Autodesk Inventor part; units mm, degrees
ref_plane "YZ Plane" through (0, 0, 0) normal (1, 0, 0) x (0, 1, 0)
ref_plane "XZ Plane" through (0, 0, 0) normal (0, 1, 0) x (-1, 0, 0)
ref_plane "XY Plane" through (0, 0, 0) normal (0, 0, 1) x (1, 0, 0)
sketch "Sketch1" plane through (0, 0, 0) normal (0, 1, 0) x (-1, 0, 0)
  circle A0 centre (0, 15.6484) radius 5.5
  line L0 (0, 15.6484) -> (0, -0.3516)
  circle A1 centre (0, -0.3516) radius 5.5
  circle A2 centre (0, 15.6484) radius 2.5
  circle A3 centre (0, -0.3516) radius 2.5
  line L1 (5.5, 15.6484) -> (5.5, -0.3516)
  line L2 (-5.5, 15.6484) -> (-5.5, -0.3516)
  point P0 (0, 0)
  dimension "d0" = 11
  dimension "d1" = 16
  dimension "d2" = 11
  dimension "d3" = 5
  dimension "d4" = 5
extrude "Extrusion1" add sketch "Sketch1" along normal blind 2
sketch "Sketch2" plane through (0, 2, 0) normal (0, 1, 0) x (1, 0, 0)
  circle A0 centre (0, -15.6484) radius 2.5
  line L0 (0, -13.1484) -> (0, -2.1484)
  circle A1 centre (0, 0.3516) radius 2.5
  line L1 (-5.5, 0.3516) -> (-5.5, -15.6484)
  line L2 (5.5, -5.6484) -> (-5.5, -5.6484)
  line L3 (-5.5, -5.6484) -> (-5.5, -9.6484)
  line L4 (-5.5, -9.6484) -> (5.5, -9.6484)
  line L5 (5.5, -9.6484) -> (5.5, -5.6484)
  line L6 (5.5, -5.6484) -> (-5.5, -9.6484) construction
  line L7 (-5.5, -5.6484) -> (5.5, -9.6484) construction
  point P0 (0, 0)
  point P1 (0, -7.6484)
  dimension "d7" = 4
extrude "Extrusion2" add sketch "Sketch2" along normal blind 4 contours L4 L1 L2 L0 | L0 L2 L5 L4
sketch "Sketch3" plane through (0, 6, 0) normal (0, 1, 0) x (1, 0, 0)
  line L0 (5.5, -5.6484) -> (-5.5, -5.6484)
  line L1 (-5.5, -5.6484) -> (-5.5, -9.6484)
  line L2 (-5.5, -9.6484) -> (5.5, -9.6484)
  line L3 (5.5, -9.6484) -> (5.5, -5.6484)
  circle A0 centre (0, -7.6484) radius 1.5
  point P0 (0, 0)
  point P1 (0, -5.3984)
  dimension "d15" = 3
extrude "Extrusion3" cut sketch "Sketch3" against normal blind 16.6375 contours A0
properties part number "bearing plate"
Read the model definition and answer for the solid it produces. Units are mm, in the model's axes. A direction names the side the tool comes from. Give positions to 0.01 mm unless a question says otherwise; leave off trailing zeros. Write each loop counter-clockwise with the first axis right and the second up, starting at its lowest first coordinate (ties: lowest second). Pieces come first, ordered by that corner, then holes. Notation, with made-up numbers: (-33, 18.5) -> (26, 18.5) arc R15 cw to (26, 36.5) -> close; hole circle Ø1 at (28, 79). An arc over 180 degrees is marked (long way). Answer as a JSON object with one key per item and string values. Group by question number.
1) Find section A-A (x = 0). Write down the section's boundary in (y, z), and give its area (3 significant figures).
2) Find section C-C (y = 1.7). Write down the section's boundary in (x, z), and give its area (3 significant figures).
3) Consider L1, parallel to Z at x = 0, y = 0.4; L2, parallel to Z at x = -2, y = 4.85; L3, parallel to Y at x = -3.75, z = 18. Determine where each line is inside the solid, lowest interval first. Write a range as from..to.
4) A tool of negligible diameter and unlimited length cuts with its end or side. For faces 5 (the cylindrical face through (0.121, 0.986, 21.147)), 6 (the flat face through (0.1, 2, 12.9)), from which of +Z, -Z, +X, -X, +Y, -Y can it reach the whole face along a straight path? Write none if from no direction.
5) Each of these flat-tipped pins is pushed along its axis until it touches: P1, Ø1.5, axis at x = -4.5, y = 2.5, coming from the +Z side; P2, Ø6, axis at x = -2.5, z = -0.5, coming from the -Y side; P3, Ø1.2, axis at x = 1, y = 4, coming from the -Z side; P4, Ø1.5, axis at x = -2.5, y = 3.5, coming from the +Z side. Where does it stop, or does it pass through?
6) The mould has two halves that part along Z. Classify faces 1 (the cylindrical face through (0.54, 0.99, 18.09)), 2 (the cylindrical face through (0.54, 0.99, 2.09)), 3 (the flat face through (0, 4, 5.648)), 4 (the flat face through (0, 2, 3)): +Z half, -Z half, draft (parallel to the pull), parting line (faces both ways), or undercut.
7) Find section D-D (x = 1.25). Write down the section's boundary in (y, z).
8) Find section B-B (z = -1.5). Write down the section's boundary in (x, y), and give its area (3 significant figures).
Values follow:
{
 "1": {"outline": "(0, -5.85) -> (2, -5.85) -> (2, -2.85) -> (0, -2.85) -> close; (0, 2.15) -> (2, 2.15) -> (2, 5.65) -> (6, 5.65) -> (6, 6.15) -> (0, 6.15) -> close; (0, 9.15) -> (6, 9.15) -> (6, 9.65) -> (2, 9.65) -> (2, 13.15) -> (0, 13.15) -> close; (0, 18.15) -> (2, 18.15) -> (2, 21.15) -> (0, 21.15) -> close", "area": "32.0 mm2"},
 "2": {"outline": "(-5.5, -0.35) arc R5.5 ccw to (5.5, -0.35) -> (5.5, 15.65) arc R5.5 ccw to (-5.5, 15.65) -> close; hole circle Ø5 at (0, -0.35); hole circle Ø5 at (0, 15.65); hole circle Ø3 at (0, 7.65)", "area": "225 mm2"},
 "3": {"L1": "z = -5.85..-2.85, 2.15..6.15, 9.15..13.15, 18.15..21.15", "L2": "z = 5.65..9.65", "L3": "y = 0..2"},
 "4": {"face 5": "+Z, +Y, -Y", "face 6": "+Z, +X, -X, +Y"},
 "5": {"P1": "stops at z = 19.48", "P2": "stops at y = 0", "P3": "stops at z = 5.65", "P4": "stops at z = 9.65"},
 "6": {"face 1": "undercut", "face 2": "undercut", "face 3": "-Z half", "face 4": "draft"},
 "7": {"outline": "(0, -5.71) -> (2, -5.71) -> (2, -2.52) -> (0, -2.52) -> close; (0, 1.81) -> (2, 1.81) -> (2, 5.65) -> (6, 5.65) -> (6, 6.82) -> (0, 6.82) -> close; (0, 8.48) -> (6, 8.48) -> (6, 9.65) -> (2, 9.65) -> (2, 13.48) -> (0, 13.48) -> close; (0, 17.81) -> (2, 17.81) -> (2, 21) -> (0, 21) -> close"},
 "8": {"outline": "(-5.38, 0) -> (-2.22, 0) -> (-2.22, 2) -> (-5.38, 2) -> close; (2.22, 0) -> (5.38, 0) -> (5.38, 2) -> (2.22, 2) -> close", "area": "12.6 mm2"}
}
